CAD build for the part. Positions are in the model's coordinates, mm. A direction names the side the tool comes from. Coordinates: 2 decimals unless noted, no trailing zeros. Loops run counter-clockwise (first coordinate to the right, second up) from the corner with the lowest first, then second, coordinate; pieces in that order, holes last.
1) Pin check, flat tips, straight feed: pin 1 Ø10 at (x, y) = (0, -31.75) entering from +Z; pin 2 Ø5.5 at (x, y) = (-0.5, -28) entering from +Z; pin 3 Ø8 at (y, z) = (25, -77) entering from +X. Stop position of each tip, or through.
2) Saw through at B-B, the plane z = -46. Write the cut outline in (x, y) (3 decimals), and give its area (3 significant figures).
3) Two-plate mould, pull along Y, no slides. Class faces 1 (the flat face through (-4, 31, -109.22)), 2 (the cylindrical face through (-0.744, -37.416, -105.463)): +Y half, -Y half, draft (parallel to the pull), parting line (faces both ways), or undercut.
4) Wall check: line 1 along Y through (x, z) = (0.25, -70.5); line 2 along Y through (x, z) = (-0.5, 17.5); line 3 along Z through (x, y) = (8.25, -32). Give the ranges that are in metal, low to high.
5) Which spindle directions (+Z, -Z, +X, -X, +Y, -Y) get a long thin tool onto all of the face, cutting with end or side? Do faces 3 (the cylindrical face through (-0.744, -37.416, -50.223)), 4 (the flat face through (4, -33, -109.22)), 5 (the cylindrical face through (-1.157, -22.936, -100.348)). Say none if no direction does.
6) Saw through at A-A, the plane x = 0. Write the cut outline in (y, z) (3 decimals).
7) Saw through at C-C, the plane z = 19.5. Give the number of separate pieces and of enclosed holes in the cut face, and give its area (3 significant figures).
```python
from build123d import *

# Parameters (mm, degrees)
F1_R     = 5.715
F1_R_2   = 3.81
F4_R     = 8.89
F4_R_2   = 4.360362463
F5_DEPTH = 2.54


with BuildPart() as f2:
    # F2: sweep along a path in F0
    with BuildLine(Plane.YZ) as f2_path:
        Line((31.75, -109.22), (31.75, 0))
        ThreePointArc((31.75, 0), (0, 31.75), (-31.75, 0))
        Line((-31.75, 0), (-31.75, -109.22))
    # F1 (on Top) → F2 (sweep)
    with BuildSketch(Plane.XY):
        with Locations((0, -31.75)):
            Circle(F1_R)
        with Locations((0, -31.75)):
            Circle(F1_R_2, mode=Mode.SUBTRACT)
    sweep(path=f2_path.line)

    # F4 (on offset) → F5 (join)
    with BuildSketch(Plane.XY.offset(-101.6)):
        with Locations((0, -31.75)):
            Circle(F4_R)
        with Locations((0, -31.75)):
            Circle(F4_R_2, mode=Mode.SUBTRACT)
    extrude(amount=F5_DEPTH)


solid = f2.part
```
Data:
1. pin 1: stops at z = 26.23
1. pin 2: stops at z = 27.66
1. pin 3: stops at x = 5.01
2. outline: circle Ø11.43 at (0, -31.75); circle Ø11.43 at (0, 31.75); hole circle Ø7.62 at (0, -31.75); hole circle Ø7.62 at (0, 31.75)
2. area: 114 mm2
3. face 1: draft
3. face 2: undercut
4. line 1: y = -37.46 to -35.55, -27.95 to -26.04, 26.04 to 27.95, 35.55 to 37.46
4. line 2: y = -33.1 to -30.92, -21.82 to -19.31, 19.31 to 21.82, 30.92 to 33.1
4. line 3: z = -101.6 to -99.06
5. face 3: none
5. face 4: -Z, +X, -X, +Y, -Y
5. face 5: -Z
6. outline: (-40.64, -101.6) - (-37.465, -101.6) - (-37.465, -109.22) - (-35.56, -109.22) - (-35.56, 0) arc R35.56 cw to (35.56, 0) - (35.56, -109.22) - (37.465, -109.22) - (37.465, 0) arc R37.465 ccw to (-37.465, 0) - (-37.465, -99.06) - (-40.64, -99.06) - close; (-27.94, -109.22) - (-26.035, -109.22) - (-26.035, -101.6) - (-22.86, -101.6) - (-22.86, -99.06) - (-26.035, -99.06) - (-26.035, 0) arc R26.035 cw to (26.035, 0) - (26.035, -109.22) - (27.94, -109.22) - (27.94, 0) arc R27.94 ccw to (-27.94, 0) - close
7. separate pieces: 2
7. enclosed holes: 2
7. area: 147 mm2
